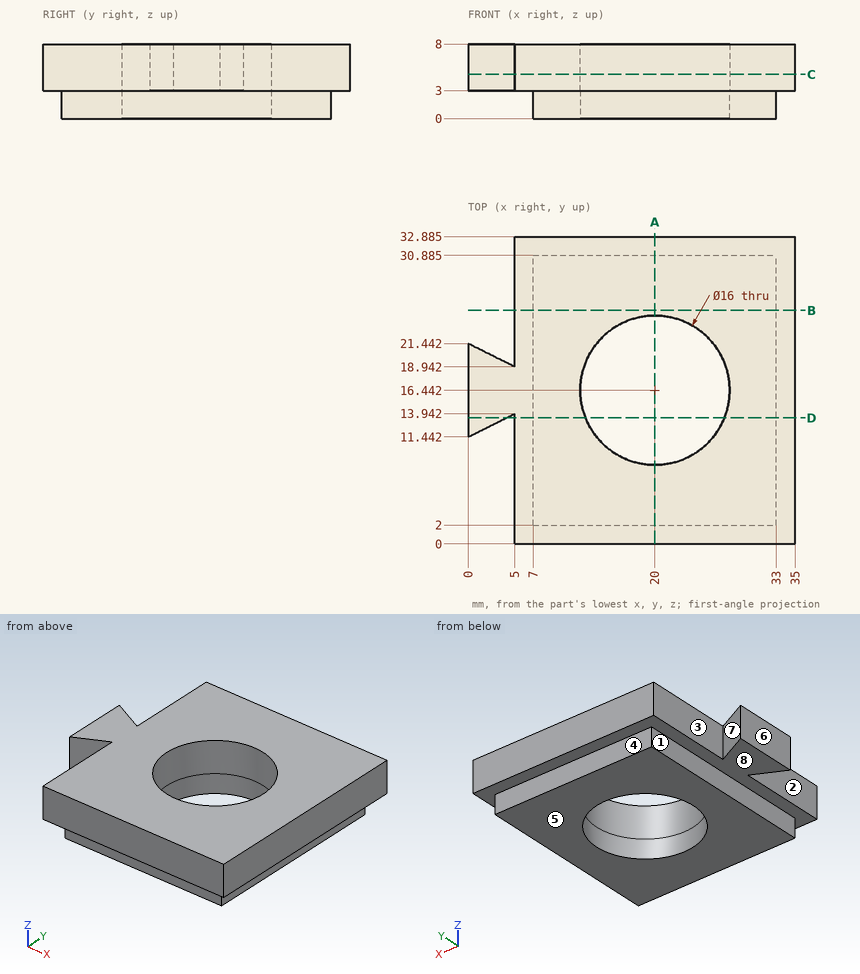
The figure shows three views and two pictorial views of one solid part (mm, origin at its lowest corner). Answer the questions. A direction names the side the tool comes from. Round coordinates to 2 decimals unless told otherwise and drop trailing zeros. Loops run counter-clockwise (first coordinate to the right, second up) from the corner with the lowest first, then second, coordinate; pieces in that order, holes last. Notation, with made-up numbers: M -33.5,66.5 L -22.5,66.5 A13 cw -22.5,88.5 Z; hole C 32.5,1 d1. An arc over 180 degrees is marked long. Return JSON: item names as keys, results as strings.
Q1. Find the intervals of material crossed by line 1 along Y through (x, z) = (20, 1.85) (1 decimal); line 2 along X through (y, z) = (12.5, 6.75) (1 decimal); line 3 along Y through (x, z) = (20, 5.8) (1 decimal), in increasing order. Write a range as from..to.
Results list:
{"line 1": "y = 2..8.4, 24.4..30.9", "line 2": "x = 0..2.1, 5..13, 27..35", "line 3": "y = 0..8.4, 24.4..32.9"}
Q2. Find section C-C, the plane z = 4.75. Determine the outline of the cut face in (x, y) (1 decimal).
Results list:
{"outline": "M 0,11.4 L 5,13.9 L 5,0 L 35,0 L 35,32.9 L 5,32.9 L 5,18.9 L 0,21.4 Z; hole C 20,16.4 d16"}
Q3. Find section B-B, the plane y = 25. Determine the outline of the cut face in (x, z).
Results list:
{"outline": "M 5,3 L 7,3 L 7,0 L 33,0 L 33,3 L 35,3 L 35,8 L 5,8 Z"}
Q4. Which of the six approach directions +Z, -Z, +X, -X, +Y, -Y give full straight-line access (tool end or side, diameter ignored) to the marked faces 1, 2, 3, 4 and 5?
Results list:
{"face 1": "-Z, -X, +Y, -Y", "face 2": "+Z, -Z, -Y", "face 3": "+Z, -Z, +Y", "face 4": "-Z, +X, -X, +Y", "face 5": "-Z, +X, -X, +Y, -Y"}
Q5. Find section A-A, the plane x = 20. Determine the outline of the cut face in (y, z) (1 decimal), plus the area to 3 significant figures.
Results list:
{"outline": "M 0,3 L 2,3 L 2,0 L 8.4,0 L 8.4,8 L 0,8 Z; M 24.4,0 L 30.9,0 L 30.9,3 L 32.9,3 L 32.9,8 L 24.4,8 Z", "area": "123 mm2"}
Q6. The mould has two halves that part along X. Classify the marked faces 6, 7 and 8: released by +X, released by -X, zero draft, split by the parting line, or undercut.
Results list:
{"face 6": "released by -X", "face 7": "undercut", "face 8": "zero draft"}
Q7. Find section D-D, the plane y = 13.5. Determine the outline of the cut face in (x, z) (1 decimal).
Results list:
{"outline": "M 0,3 L 4.1,3 L 4.1,8 L 0,8 Z; M 5,3 L 7,3 L 7,0 L 12.6,0 L 12.6,8 L 5,8 Z; M 27.4,0 L 33,0 L 33,3 L 35,3 L 35,8 L 27.4,8 Z"}
Q8. Each of these flat-tipped pins is pushed along its axis until it touches: pin 1 Ø2.5 at (x, z) = (19, 1) entering from -Y; pin 2 Ø3.5 at (y, z) = (17, 2) entering from -X; pin 3 Ø13 at (x, y) = (20, 16.44) entering from +Z; pin 4 Ø1.5 at (x, z) = (24.5, 2) entering from +Y (1 decimal). Where does it stop, or does it pass through?
Results list:
{"pin 1": "stops at y = 2", "pin 2": "stops at x = 0", "pin 3": "passes through", "pin 4": "stops at y = 30.9"}
